The listing builds one solid part. Answer for the finished solid, in the listing's coordinates (mm). Face numbers are marked on the shaded views. A direction names the side the tool comes from. Give positions to 0.01 mm unless a question says otherwise; leave off trailing zeros. Write each loop counter-clockwise with the first axis right and the second up, starting at its lowest first coordinate (ties: lowest second). Pieces come first, ordered by that corner, then holes.
```python
from build123d import *

# Parameters (mm, degrees)
BOSS_EXTRUDE1_DEPTH = 20
FILLET1_R           = 2
BOSS_EXTRUDE2_DEPTH = 0.5
CUT_EXTRUDE1_DEPTH  = 17
CUT_EXTRUDE2_DEPTH  = 3
SKETCH5_R           = 1
CUT_EXTRUDE3_DEPTH  = 10
SKETCH6_R           = 1.5
CUT_EXTRUDE4_DEPTH  = 10


with BuildPart() as part:
    # Sketch1 → Boss-Extrude1 (new body)
    with BuildSketch(Plane(origin=(0, 0, 0), x_dir=(1, 0, 0), z_dir=(0, 1, 0))):
        with BuildLine():
            Line((-41, 26.5), (41, 26.5))
            ThreePointArc((41, 26.5), (42.414213562, 25.914213562), (43, 24.5))
            Line((43, 24.5), (43, -24.5))
            ThreePointArc((43, -24.5), (42.414213562, -25.914213562), (41, -26.5))
            Line((41, -26.5), (-41, -26.5))
            ThreePointArc((-41, -26.5), (-42.414213562, -25.914213562), (-43, -24.5))
            Line((-43, -24.5), (-43, 24.5))
            ThreePointArc((-43, 24.5), (-42.414213562, 25.914213562), (-41, 26.5))
        make_face()
    extrude(amount=BOSS_EXTRUDE1_DEPTH)

    # Fillet1
    fillet1_edges = [part.edges().sort_by_distance(p)[0] for p in [
        (-42.414213562, 20, -25.914213562),
        (-43, 20, 0),
        (-42.414213562, 20, 25.914213562),
        (0, 20, 26.5),
        (42.414213562, 20, 25.914213562),
        (43, 20, 0),
        (42.414213562, 20, -25.914213562),
        (0, 20, -26.5),
    ]]
    fillet(fillet1_edges, radius=FILLET1_R)

    # Sketch2 → Boss-Extrude2 (add)
    with BuildSketch(Plane(origin=(0, 20, 0), x_dir=(1, 0, 0), z_dir=(0, 1, 0))):
        with BuildLine():
            Line((-35, 21.5), (35, 21.5))
            ThreePointArc((35, 21.5), (37.121320344, 20.621320344), (38, 18.5))
            Line((38, 18.5), (38, -18.5))
            ThreePointArc((38, -18.5), (37.121320344, -20.621320344), (35, -21.5))
            Line((35, -21.5), (-35, -21.5))
            ThreePointArc((-35, -21.5), (-37.121320344, -20.621320344), (-38, -18.5))
            Line((-38, -18.5), (-38, 18.5))
            ThreePointArc((-38, 18.5), (-37.121320344, 20.621320344), (-35, 21.5))
        make_face()
    extrude(amount=BOSS_EXTRUDE2_DEPTH)

    # Sketch3 → Cut-Extrude1 (cut)
    with BuildSketch(Plane.XZ):
        with BuildLine():
            Line((-37, 23.5), (37, 23.5))
            ThreePointArc((37, 23.5), (39.121320344, 22.621320344), (40, 20.5))
            Line((40, 20.5), (40, -20.5))
            ThreePointArc((40, -20.5), (39.121320344, -22.621320344), (37, -23.5))
            Line((37, -23.5), (-37, -23.5))
            ThreePointArc((-37, -23.5), (-39.121320344, -22.621320344), (-40, -20.5))
            Line((-40, -20.5), (-40, 20.5))
            ThreePointArc((-40, 20.5), (-39.121320344, 22.621320344), (-37, 23.5))
        make_face()
    extrude(amount=-CUT_EXTRUDE1_DEPTH, mode=Mode.SUBTRACT)

    # Sketch4 → Cut-Extrude2 (cut)
    with BuildSketch(Plane.XZ):
        with BuildLine():
            Line((38.25, -24.75), (-38.25, -24.75))
            ThreePointArc((-38.25, -24.75), (-40.371320344, -23.871320344), (-41.25, -21.75))
            Line((-41.25, -21.75), (-41.25, 21.75))
            ThreePointArc((-41.25, 21.75), (-40.371320344, 23.871320344), (-38.25, 24.75))
            Line((-38.25, 24.75), (38.25, 24.75))
            ThreePointArc((38.25, 24.75), (40.371320344, 23.871320344), (41.25, 21.75))
            Line((41.25, 21.75), (41.25, -21.75))
            ThreePointArc((41.25, -21.75), (40.371320344, -23.871320344), (38.25, -24.75))
        make_face()
    extrude(amount=-CUT_EXTRUDE2_DEPTH, mode=Mode.SUBTRACT)

    # Sketch5 → Cut-Extrude3 (cut)
    with BuildSketch(Plane(origin=(0, 20.5, 0), x_dir=(1, 0, 0), z_dir=(0, 1, 0))):
        with Locations(Location((-2.5, -5, 0), (0, 0, 270))):
            Circle(SKETCH5_R)
        with Locations(Location((2.5, -5, 0), (0, 0, 270))):
            Circle(SKETCH5_R)
    extrude(amount=-CUT_EXTRUDE3_DEPTH, mode=Mode.SUBTRACT)

    # Sketch6 → Cut-Extrude4 (cut)
    with BuildSketch(Plane(origin=(43, 0, 0), x_dir=(0, 0, -1), z_dir=(1, 0, 0))):
        with Locations((11.365424158, 6)):
            Circle(SKETCH6_R)
        with BuildLine():
            Line((17.332844904, 7.5), (11.365424158, 7.5))
            ThreePointArc((11.365424158, 7.5), (12.426084329, 7.060660172), (12.865424158, 6))
            ThreePointArc((12.865424158, 6), (12.426084329, 4.939339828), (11.365424158, 4.5))
            Line((11.365424158, 4.5), (17.332844904, 4.5))
            ThreePointArc((17.332844904, 4.5), (15.832844904, 6), (17.332844904, 7.5))
        make_face()
        with Locations((17.332844904, 6)):
            Circle(SKETCH6_R)
    extrude(amount=-CUT_EXTRUDE4_DEPTH, mode=Mode.SUBTRACT)


solid = part.part
```
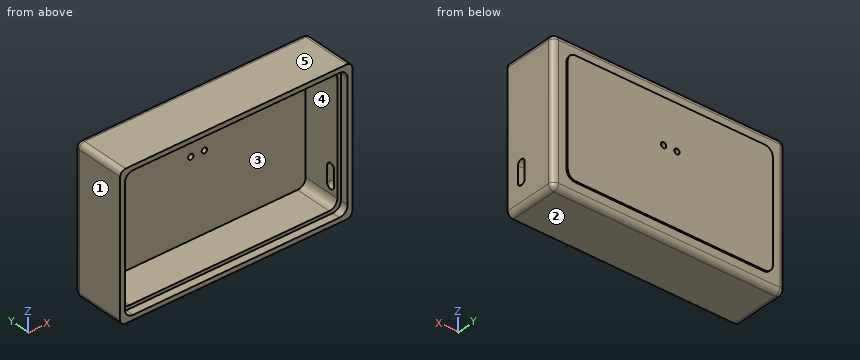
Item 1: A cutting plane is placed at A-A, the plane z = 5. Give the vertices of the cut face in (x, y), plus the area to 3 significant figures.
Conclusion:
outline: (-43, 0) - (-41.25, 0) - (-41.25, 3) - (-40, 3) - (-40, 17) - (-3.5, 17) - (-3.5, 20.5) - (-38, 20.5) - (-38, 20) - (-41, 20) arc R2 ccw to (-43, 18) - close; (-1.5, 17) - (1.5, 17) - (1.5, 20.5) - (-1.5, 20.5) - close; (3.5, 17) - (40, 17) - (40, 3) - (41.25, 3) - (41.25, 0) - (43, 0) - (43, 18) arc R2 ccw to (41, 20) - (38, 20) - (38, 20.5) - (3.5, 20.5) - close
area: 375 mm2
Item 2: Which of the six approach directions +Z, -Z, +X, -X, +Y, -Y give full straight-line access (tool end or side, diameter ignored) to the marked faces 4 and 5?
Conclusion:
face 4: -Y
face 5: +Z, +X, -X, +Y, -Y
Item 3: A cutting plane is placed at D-D, the plane z = -15.5. Give the vertices of the cut face in (x, y), plus the area to 3 significant figures.
Conclusion:
outline: (-43, 0) - (-41.25, 0) - (-41.25, 3) - (-40, 3) - (-40, 17) - (40, 17) - (40, 7.5) - (43, 7.5) - (43, 18) arc R2 ccw to (41, 20) - (38, 20) - (38, 20.5) - (-38, 20.5) - (-38, 20) - (-41, 20) arc R2 ccw to (-43, 18) - close; (40, 3) - (41.25, 3) - (41.25, 0) - (43, 0) - (43, 4.5) - (40, 4.5) - close
area: 380 mm2
Item 4: Consider probe 1 along X at (y, z) = (18.2, 5); probe 2 along X at (y, z) = (15.75, -0.5); probe 3 along Z at (x, y) = (37, 16). Determine where each line is inside the solid, lowest interval first.
Conclusion:
probe 1: x = -42.99 to -3.5, -1.5 to 1.5, 3.5 to 42.99
probe 2: x = -43 to -40, 40 to 43
probe 3: z = -26.5 to -23.5, 23.5 to 26.5
Item 5: A cutting plane is placed at C-C, the plane y = 1.75. Give the vertices of the cut face in (x, z), plus the area to 3 significant figures.
Conclusion:
outline: (-43, -24.5) arc R2 ccw to (-41, -26.5) - (41, -26.5) arc R2 ccw to (43, -24.5) - (43, 24.5) arc R2 ccw to (41, 26.5) - (-41, 26.5) arc R2 ccw to (-43, 24.5) - close; hole (-41.25, -21.75) arc R3 ccw to (-38.25, -24.75) - (38.25, -24.75) arc R3 ccw to (41.25, -21.75) - (41.25, 21.75) arc R3 ccw to (38.25, 24.75) - (-38.25, 24.75) arc R3 ccw to (-41.25, 21.75) - close
area: 479 mm2
Item 6: Each of these flat-tipped pins is pushed along its axis until it touches: P1, Ø1.8, axis at x = -2.5, z = 5, coming from the -Y side; P2, Ø12, axis at x = 26, z = 11.5, coming from the -Y side; P3, Ø0.6, axis at x = 12.5, y = 20.5, coming from the +Z side; P4, Ø3.5, axis at x = 42, z = -15.5, coming from the +Y side. Where does it stop, or does it pass through?
Conclusion:
P1: passes through
P2: stops at y = 17
P3: stops at z = 21.5
P4: stops at y = 20
Item 7: A cutting plane is placed at B-B, the plane x = 2.5. Give the vertices of the cut face in (y, z).
Conclusion:
outline: (0, -26.5) - (18, -26.5) arc R2 ccw to (20, -24.5) - (20, -21.5) - (20.5, -21.5) - (20.5, 4) - (17, 4) - (17, -23.5) - (3, -23.5) - (3, -24.75) - (0, -24.75) - close; (0, 24.75) - (3, 24.75) - (3, 23.5) - (17, 23.5) - (17, 6) - (20.5, 6) - (20.5, 21.5) - (20, 21.5) - (20, 24.5) arc R2 ccw to (18, 26.5) - (0, 26.5) - close
Item 8: Determine the mould class of the marked faces 1, 2 and 3 for opening direction X: pulls with the +X half, pulls with the -X half, needs draft (parallel to the pull), parting line crosses it, or undercut.
Conclusion:
face 1: pulls with the -X half
face 2: needs draft
face 3: undercut
